Model file for the job. Use its own axes, mm. Round coordinates to 2 decimals unless told otherwise and drop trailing zeros. Order: outer loops, then holes, each group sorted by start corner. A loop starts at its lowest first (then second) coordinate and runs counter-clockwise, first axis right, second up. Notation, with made-up numbers: (56, 66) -> (78, 66) arc R24 ccw to (78, 80) -> close; hole circle Ø9 at (-15, -14). An arc over 180 degrees is marked (long way). Answer as CSV lines item,"result".
```python
from build123d import *

# Parameters (mm, degrees)
F1_DEPTH = 12.7


with BuildPart() as f1:
    # F0 (on Front) → F1 (new body)
    with BuildSketch(Plane.XZ):
        with BuildLine():
            Line((0, 38.199143), (0, 0))
            Line((0, 0), (76.2, 0))
            Line((76.2, 0), (76.2, 38.199143))
            Line((76.2, 38.199143), (43.408294, 70.905519))
            Line((43.408294, 70.905519), (43.23573, 71.077634))
            ThreePointArc((43.23573, 71.077634), (38.1, 73.151625), (32.96427, 71.077634))
            Line((32.96427, 71.077634), (32.791706, 70.905519))
            Line((32.791706, 70.905519), (0, 38.199143))
        make_face()
        with BuildLine():
            ThreePointArc((32.96427, 71.077634), (32.877279, 70.992288), (32.791706, 70.905519))
            Line((32.791706, 70.905519), (32.96427, 71.077634))
        make_face()
        with BuildLine():
            Line((43.23573, 71.077634), (43.408294, 70.905519))
            ThreePointArc((43.408294, 70.905519), (43.322721, 70.992288), (43.23573, 71.077634))
        make_face()
    extrude(amount=F1_DEPTH)


solid = f1.part
```
Q1. Wall check: L1, parallel to X at y = -0.5, z = 65; L2, parallel to X at y = -2.25, z = 49; L3, parallel to Z at x = 29, y = -2.5. Give the ranges that are in metal, low to high. Write a range as [from, to].
Checks:
L1,"[26.87, 49.33]"
L2,"[10.83, 65.37]"
L3,"[0, 67.12]"
Q2. Saw through at A-A (y = -7). Write the cut outline in (x, z).
Checks:
outline,"(0, 0) -> (76.2, 0) -> (76.2, 38.2) -> (43.41, 70.91) arc R7.39 ccw to (43.24, 71.08) arc R7.4 ccw to (32.96, 71.08) arc R7.39 ccw to (32.79, 70.91) -> (0, 38.2) -> close"
Q3. Flat gauge pins, fed straight in: pin 1 (1.5 mm diameter, centred on y = -6, z = 55, fed in from -X); pin 2 (1 mm diameter, centred on x = 34.5, y = -1.5, fed in from -Z); pin 3 (5 mm diameter, centred on x = 43.5, y = -7, fed in from +Z). Where does each tip first touch, or does it go through?
Checks:
pin 1,"x = 16.09"
pin 2,"z = 0"
pin 3,"z = 72.56"
Q4. Saw through at C-C (z = 54.5). Write the cut outline in (x, y).
Checks:
outline,"(16.34, -12.7) -> (59.86, -12.7) -> (59.86, 0) -> (16.34, 0) -> close"
Q5. Saw through at B-B (x = 48.5). Write the cut outline in (y, z).
Checks:
outline,"(-12.7, 0) -> (0, 0) -> (0, 65.83) -> (-12.7, 65.83) -> close"
